from build123d import *


with BuildPart() as part:
    # 草图2 → Revolve 706 (revolve)
    with BuildSketch(Plane.XY, mode=Mode.PRIVATE) as revolve_706_sk:
        with BuildLine():
            Line((0, 0), (17.1, 0))
            Line((17.1, 0), (17.1, 2))
            Line((17.1, 2), (4.5, 2))
            Line((4.5, 2), (4.232, 1.732))
            Line((4.232, 1.732), (3.718, 1.732))
            ThreePointArc((3.718, 1.732), (3.281008009, 1.913008009), (3.1, 2.35))
            Line((3.1, 2.35), (3.1, 4))
            Line((3.1, 4), (1.376524617, 4))
            ThreePointArc((1.376524617, 4), (0.353757652, 2.115113473), (0, 0))
        make_face()
    revolve(revolve_706_sk.sketch.rotate(Axis((-1.331757704, 0, 0), (1, 0, 0)), 90), axis=Axis((-1.331757704, 0, 0), (1, 0, 0)))

    # 草图3 → 切除-旋转1 (revolve, cut)
    with BuildSketch(Plane.XY, mode=Mode.PRIVATE) as cut_revolve_1_sk:
        Polygon((16.753791204, 2), (17.453791204, 2), (17.1, 1.3938), align=None)
    revolve(cut_revolve_1_sk.sketch.rotate(Axis((-0.242766179, 0, 0), (1, 0, 0)), 90), axis=Axis((-0.242766179, 0, 0), (1, 0, 0)), mode=Mode.SUBTRACT)

    # 草图5 → 切除-放样1 section 0
    with BuildSketch(Plane(origin=(0, 0, 0), x_dir=(0, 0, -1), z_dir=(1, 0, 0)), mode=Mode.PRIVATE) as loft_1_s0:
        with BuildLine():
            Line((0.35, 2.2), (-0.35, 2.2))
            Line((-0.35, 2.2), (-0.35, -2.2))
            Line((-0.35, -2.2), (0.35, -2.2))
            Line((0.35, -2.2), (0.35, 2.2))
        make_face()
    loft_1 = loft([Vertex(2.4, 0, 0), loft_1_s0.sketch], mode=Mode.SUBTRACT)

    # 镜向1: 切除-放样1 across plane
    add(loft_1.mirror(Plane(origin=(0, 0, 0), x_dir=(0, 0.7071067811865462, 0.7071067811865488), z_dir=(0, -0.7071067811865488, 0.7071067811865462))), mode=Mode.SUBTRACT)


solid = part.part
Part model, mm, in its own coordinate system. A direction names the side the tool comes from. Give positions to 0.01 mm unless a question says otherwise; leave off trailing zeros. Order: outer loops, then holes, each group sorted by start corner. A loop starts at its lowest first (then second) coordinate and runs counter-clockwise, first axis right, second up. Notation, with made-up numbers: (80, 8) - (138, 8) arc R10 ccw to (138, 27) - close; hole circle Ø3 at (-25, 40.5). An arc over 180 degrees is marked (long way). One line per question, with ' | ' between items.
1. Band-saw the part on A-A on y = 3.25. List the corners of the cut face in (x, z), then the cut area to 3 significant figures.
Filled in:
outline: (1.38, -2.33) - (3.1, -2.33) - (3.1, 2.33) - (1.38, 2.33) arc R5.63 ccw to start | area: 9.62 mm²
2. Drop flat-ended pins along their axis: P1, Ø2, axis at x = 3.5, z = -0.5, coming from the +Y side; P2, Ø1.5, axis at y = 3, z = 0, coming from the +X side. Give the stop position or say it passes through.
Filled in:
P1: y = 4 | P2: x = 3.11
3. Which spindle directions (+Z, -Z, +X, -X, +Y, -Y) get a long thin tool onto all of the face, cutting with end or side? Do faces 1 (the face through (3.1, 2, -2)), 2 (the face through (3.97, -0.52, 1.65)), 3 (the face through (0.928, -0.735, 0.215)). Say none if no direction does.
Filled in:
face 1: +X | face 2: none | face 3: -X
4. Band-saw the part on B-B on z = -3. List the corners of the cut face in (x, y).
Filled in:
outline: (1.38, -2.65) - (3.1, -2.65) - (3.1, 2.65) - (1.38, 2.65) arc R5.77 ccw to start
5. Pull direction Y, two halves, no side cores. Call faces 4 (the face through (11, 2, 0)), 5 (the face through (1.1, 1.19, 0)), 6 (the face through (0.928, 0.215, 0.762)), 7 (the face through (17.1, 0, 0)): +Y half, -Y half, draft (parallel to the pull), parting line (faces both ways), or undercut.
Filled in:
face 4: parting line | face 5: undercut | face 6: undercut | face 7: draft
6. Drill centre lines: probe 1 along Y at (x, z) = (6.75, -1); probe 2 along X at (y, z) = (3.75, 1); probe 3 along Y at (x, z) = (11, -1.25). Where is each one in solid material? Low to high.
Filled in:
probe 1: -1.73 to 1.73 | probe 2: 1.29 to 3.1 | probe 3: -1.56 to 1.56
